Model file for the job. Use its own axes, mm. Face numbers are marked on the shaded views. A direction names the side the tool comes from. Coordinates: 2 decimals unless noted, no trailing zeros. Write each loop counter-clockwise with the first axis right and the second up, starting at its lowest first coordinate (ties: lowest second). Pieces come first, ordered by that corner, then holes.
Q1. Band-saw the part on D-D, the plane z = 5.5. Write the cut outline in (x, y).
Q2. Band-saw the part on B-B, the plane z = 7.5. Write the cut outline in (x, y), plus the area to 3 significant figures.
Q3. Band-saw the part on A-A, the plane x = 0. Write the cut outline in (y, z), plus the area to 3 significant figures.
Q4. Drill centre lines: probe 1 along Z at (x, y) = (0.5, 3.75); probe 2 along Y at (x, z) = (1, 8.25); probe 3 along X at (y, z) = (1, 4). Where is each one in solid material? Low to high.
Q5. Which spindle directions (+Z, -Z, +X, -X, +Y, -Y) get a long thin tool onto all of the face, cutting with end or side? Do the marked faces 1, 2 and 3. Say none if no direction does.
Q6. Band-saw the part on C-C, the plane y = 1.5. Write the cut outline in (x, z), plus the area to 3 significant figures.
Q7. Pin check, flat tips, straight feed: P1, Ø0.5, axis at x = 1.5, z = 8.5, coming from the +Y side; P2, Ø1.5, axis at x = 3.5, y = -3.5, coming from the +Z side; P3, Ø3.5, axis at y = 2, z = 5, coming from the -X side. Stop position of each tip, or through.
Q8. Pull direction X, two halves, no side cores. Call the marked faces 4, 5 and 6: released by +X, released by -X, zero draft, split by the parting line, or undercut.
from build123d import *

# Parameters (mm, degrees)
STOCK_5_GEAR_5_OUTPUT_GEAR_32TEETH_0_5M_DEPTH = 6
STOCK_5_GEAR_START                            = 6
STOCK_5_GEAR_5_OUTPUT_GEAR_32TEETH_3_DEPTH    = 5
SKETCH1_W                                     = 2.3
SKETCH1_H                                     = 6.8
BOSS_EXTRUDE1_DEPTH                           = 4
BOSS_EXTRUDE1_DRAFT                           = 1
SKETCH1_W_2                                   = 4.8
SKETCH1_H_2                                   = 2.3
BOSS_EXTRUDE1_PROFILE_2_DEPTH                 = 4
BOSS_EXTRUDE1_PROFILE_2_DRAFT                 = 1
SKETCH2_R                                     = 5
BOSS_EXTRUDE2_DEPTH                           = 1


# Read off the part's stored shape, not the designer's step: Stock-5_Gear 5__Output Gear_32Teeth_0.5Modulus-1
with BuildPart() as part:
    # Stock-5_Gear 5__Output Gear_32Teeth_ 2 → Stock-5_Gear 5__Output Gear_32Teeth_0.5Modulus-1 (new body)
    with BuildSketch(Plane.XY):
        with BuildLine():
            ThreePointArc((-0.75, 3.16227766), (0, -3.25), (0.75, 3.16227766))
            Line((0.75, 3.16227766), (0.75, 0))
            ThreePointArc((0.75, 0), (0, -0.75), (-0.75, 0))
            Line((-0.75, 0), (-0.75, 3.16227766))
        make_face()
    extrude(amount=STOCK_5_GEAR_5_OUTPUT_GEAR_32TEETH_0_5M_DEPTH)

    # Stock-5_Gear 5__Output Gear_32Teeth_ 3 o → Stock-5_Gear 5__Output Gear_32Teeth_ 3 (add)
    with BuildSketch(Plane.XY.offset(STOCK_5_GEAR_START)):
        with BuildLine():
            Line((1.674066904, 1), (0.75, 1))
            Line((0.75, 1), (0.75, 0))
            ThreePointArc((0.75, 0), (0, -0.75), (-0.75, 0))
            Line((-0.75, 0), (-0.75, 1))
            Line((-0.75, 1), (-1.674066904, 1))
            ThreePointArc((-1.674066904, 1), (0, -1.95), (1.674066904, 1))
        make_face()
    extrude(amount=STOCK_5_GEAR_5_OUTPUT_GEAR_32TEETH_3_DEPTH)


with BuildPart() as boss_extrude1_tool:
    # Sketch1 → Boss-Extrude1 (with draft: the straight prism first)
    with BuildSketch(Plane(origin=(0, 0, 0), x_dir=(-1, 0, 0), z_dir=(0, 0, -1))):
        Rectangle(SKETCH1_W, SKETCH1_H)
    extrude(amount=BOSS_EXTRUDE1_DEPTH)
    # Boss-Extrude1: the draft: its side faces are tilted about the plane it starts from
    boss_extrude1_sides = [boss_extrude1_tool.faces().sort_by_distance(p)[0] for p in [
        (0, -3.4, -2),
        (-1.15, 0, -2),
        (0, 3.4, -2),
        (1.15, 0, -2),
    ]]
    draft(boss_extrude1_sides, Plane(origin=(0, 0, 0), x_dir=(-1, 0, 0), z_dir=(0, 0, -1)), BOSS_EXTRUDE1_DRAFT)


with BuildPart() as part_1:
    add(part.part)

    # Boss-Extrude1: add boss_extrude1_tool
    add(boss_extrude1_tool.part)


with BuildPart() as boss_extrude1_profile_2_tool:
    # Sketch1 → Boss-Extrude1 profile 2 (with draft: the straight prism first)
    with BuildSketch(Plane(origin=(0, 0, 0), x_dir=(-1, 0, 0), z_dir=(0, 0, -1))):
        with Locations((0, 2.25)):
            Rectangle(SKETCH1_W_2, SKETCH1_H_2)
    extrude(amount=BOSS_EXTRUDE1_PROFILE_2_DEPTH)
    # Boss-Extrude1 profile 2: the draft: its side faces are tilted about the plane it starts from
    boss_extrude1_profile_2_sides = [boss_extrude1_profile_2_tool.faces().sort_by_distance(p)[0] for p in [
        (0, 3.4, -2),
        (2.4, 2.25, -2),
        (0, 1.1, -2),
        (-2.4, 2.25, -2),
    ]]
    draft(boss_extrude1_profile_2_sides, Plane(origin=(0, 0, 0), x_dir=(-1, 0, 0), z_dir=(0, 0, -1)), BOSS_EXTRUDE1_PROFILE_2_DRAFT)


with BuildPart() as part_2:
    add(part_1.part)

    # Boss-Extrude1 profile 2: add boss_extrude1_profile_2_tool
    add(boss_extrude1_profile_2_tool.part)

    # Sketch2 → Boss-Extrude2 (add)
    with BuildSketch(Plane(origin=(0, 0, 0), x_dir=(-1, 0, 0), z_dir=(0, 0, -1))):
        Circle(SKETCH2_R)
    extrude(amount=BOSS_EXTRUDE2_DEPTH)


solid = part_2.part
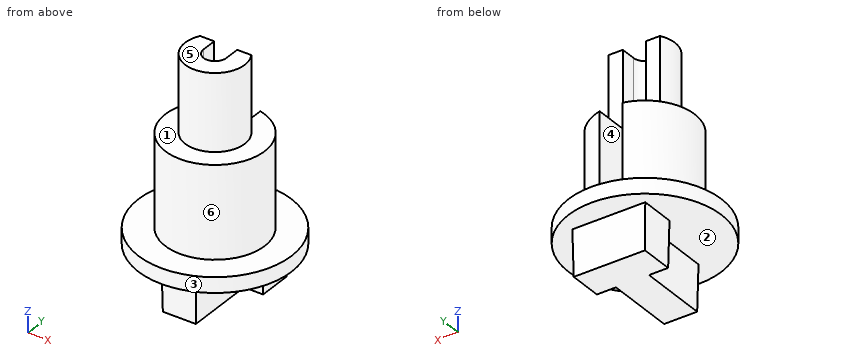
Answer sheet:
1. outline: (-0.75, 0) - (-0.75, 3.16) arc R3.25 ccw (long way) to (0.75, 3.16) - (0.75, 0) arc R0.75 cw to start
2. outline: (-1.67, 1) arc R1.95 ccw (long way) to (1.67, 1) - (0.75, 1) - (0.75, 0) arc R0.75 cw to (-0.75, 0) - (-0.75, 1) - close
2. area: 7.31 mm2
3. outline: (-5, -1) - (-3.38, -1) - (-3.33, -4) - (3.33, -4) - (3.38, -1) - (5, -1) - (5, 0) - (-0.75, 0) - (-0.75, 11) - (-1.95, 11) - (-1.95, 6) - (-3.25, 6) - (-3.25, 0) - (-5, 0) - close
3. area: 51.1 mm2
4. probe 1: z = -1 to 0
4. probe 2: y = -1.67 to 1
4. probe 3: x = -3.09 to -0.75, 0.75 to 3.09
5. face 1: +Z
5. face 2: -Z
5. face 3: +Z, -Z
6. outline: (-4.77, -1) - (-2.38, -1) - (-2.33, -4) - (2.33, -4) - (2.38, -1) - (4.77, -1) - (4.77, 0) - (2.88, 0) - (2.88, 6) - (0.75, 6) - (0.75, 0) - (-0.75, 0) - (-0.75, 6) - (-2.88, 6) - (-2.88, 0) - (-4.77, 0) - close
6. area: 49.3 mm2
7. P1: stops at y = 1
7. P2: stops at z = 0
7. P3: stops at x = -3.24
8. face 4: undercut
8. face 5: zero draft
8. face 6: split by the parting line
